Verification items for this drawing (mm, ordinates from the low corner). Round coordinates to 2 decimals unless told otherwise and drop trailing zeros. Loops run counter-clockwise (first coordinate to the right, second up) from the corner with the lowest first, then second, coordinate; pieces in that order, holes last. Notation, with made-up numbers: (-6.75, 64) - (30.25, 64) arc R15 cw to (30.25, 83) - close; hole circle Ø8 at (56, 79.25). An arc over 180 degrees is marked (long way). Put each result on its own line as item: value.
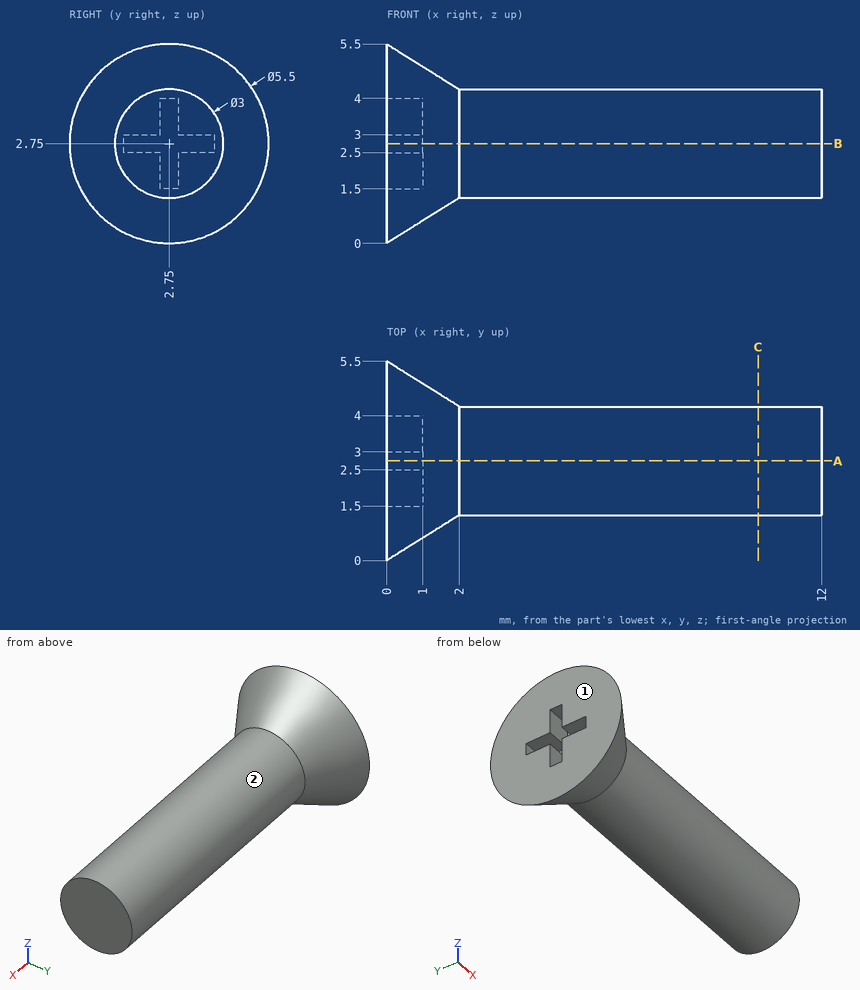
Item 1: Go/stop test with flat-tipped pins: pin 1 (0.8 mm diameter, centred on x = 0.5, y = 2, fed in from +Z); pin 2 (1 mm diameter, centred on x = 8.5, z = 1.5, fed in from -Y); pin 3 (0.5 mm diameter, centred on x = 0.5, z = 2, fed in from -Y). Record where each tip stops, or that it passes through.
Filled sheet:
pin 1: z = 5.35
pin 2: y = 1.45
pin 3: y = 0.25
Item 2: Thickness scan on line 1 (Y direction, x = 2.5, z = 2.7); line 2 (Z direction, x = 11, y = 4); line 3 (X direction, y = 4.8, z = 4.05). Record the ranges inside material, lowest first. Write a range as from..to.
Filled sheet:
line 1: 1.25..4.25
line 2: 1.92..3.58
line 3: 0..0.52
Item 3: Release check for a two-part mould opening along Y. For the marked faces 1 and 2 record: +Y half, -Y half, draft (parallel to the pull), parting line (faces both ways), or undercut.
Filled sheet:
face 1: draft
face 2: parting line
Item 4: Section check A-A on y = 2.75. Enter the section's corners in (x, z), then the cut area to 3 significant figures.
Filled sheet:
outline: (0, 0) - (2, 1.25) - (12, 1.25) - (12, 4.25) - (2, 4.25) - (0, 5.5) - (0, 4) - (1, 4) - (1, 1.5) - (0, 1.5) - close
area: 36.0 mm²
Item 5: Section check C-C on x = 10.25. Enter the section's corners in (y, z), then the cut area to 3 significant figures.
Filled sheet:
outline: circle Ø3 at (2.75, 2.75)
area: 7.07 mm²
